```python
from build123d import *

# Parameters (mm, degrees)
SKETCH1_W               = 19.05
SKETCH1_H               = 19.05
SKETCH1_W_2             = 15.875
SKETCH1_H_2             = 15.875
BOSS_EXTRUDE1_DEPTH     = 196.85
CUT_EXTRUDE1_DEPTH      = 198.310348816
CUT_EXTRUDE1_DEPTH_BACK = 198.310348816
SKETCH2_R               = 6.35
SKETCH3_R               = 2.5
CUT_EXTRUDE2_DEPTH      = 30
SKETCH4_R               = 2.38125
CUT_EXTRUDE3_DEPTH      = 30


with BuildPart() as part:
    # Sketch1 → Boss-Extrude1 (new, symmetric)
    with BuildSketch(Plane.XY):
        Rectangle(SKETCH1_W, SKETCH1_H)
        Rectangle(SKETCH1_W_2, SKETCH1_H_2, mode=Mode.SUBTRACT)
    extrude(amount=BOSS_EXTRUDE1_DEPTH, both=True)

    # Sketch2 → Cut-Extrude1 (cut, two sides: drawn at the far end of the back side and taken through both)
    with BuildSketch(Plane(origin=(0, 0, 0), x_dir=(0, 0, -1), z_dir=(1, 0, 0)).offset(-CUT_EXTRUDE1_DEPTH_BACK)):
        Circle(SKETCH2_R)
    extrude(amount=CUT_EXTRUDE1_DEPTH + CUT_EXTRUDE1_DEPTH_BACK, mode=Mode.SUBTRACT)

    # Sketch3 → Cut-Extrude2 (cut)
    with BuildSketch(Plane(origin=(-152.4, 13.525, 0), x_dir=(1, 0, 0), z_dir=(0, 1, 0))):
        with Locations(Location((152.4, -186.375, 0), (0, 0, 270))):
            Circle(SKETCH3_R)
        with Locations(Location((152.4, -166.375, 0), (0, 0, 270))):
            Circle(SKETCH3_R)
    cut_extrude2 = extrude(amount=-CUT_EXTRUDE2_DEPTH, mode=Mode.SUBTRACT)

    # Mirror1: Cut-Extrude2 across Front Plane
    add(cut_extrude2.mirror(Plane.XY), mode=Mode.SUBTRACT)

    # Sketch4 → Cut-Extrude3 (cut)
    with BuildSketch(Plane(origin=(-152.4, 18.1864, 0), x_dir=(1, 0, 0), z_dir=(0, 1, 0))):
        with Locations(Location((152.4, -127, 0), (0, 0, 270))):
            Circle(SKETCH4_R)
        with Locations(Location((152.4, 127, 0), (0, 0, 270))):
            Circle(SKETCH4_R)
        with Locations(Location((152.4, -50.8, 0), (0, 0, 270))):
            Circle(SKETCH4_R)
        with Locations(Location((152.4, 50.8, 0), (0, 0, 270))):
            Circle(SKETCH4_R)
    extrude(amount=-CUT_EXTRUDE3_DEPTH, mode=Mode.SUBTRACT)


solid = part.part
```
Input: part model. Units: mm. Frame: model coordinates. A direction names the side the tool comes from. Coordinates: 2 decimals unless noted, no trailing zeros.
Q1. Mould query, pull axis Y, two halves, no side actions, for faces 1 (the flat face through (9.525, 6, 3)), 2 (the flat face through (0, 9.525, 3)), 3 (the cylindrical face through (8.72, -6.2, 1.38)). Classes: +Y half, -Y half, draft (parallel to the pull), parting line (faces both ways), or undercut.
Results are:
face 1: draft
face 2: +Y half
face 3: undercut
Q2. Contact query for a flat-ended pin moving along its axis: pin 1 (3 mm diameter, centred on x = 0, z = -166.375, fed in from -Y). Output: stop coordinate, or through.
Results are:
pin 1: passes through
Q3. Line query: line 1 along X through (y, z) = (-5.25, 98.5) (1 decimal); line 2 along X through (y, z) = (-8.4, 127) (3 decimals). Output: solid intervals per line, ascending.
Results are:
line 1: x = -9.5 to -7.9, 7.9 to 9.5
line 2: x = -9.525 to -2.381, 2.381 to 9.525
Q4. Set-up query: faces 4 (the flat face through (-7.938, 7, 3)), 5 (the flat face through (-9, 0, -196.85)). Return all of +Z, -Z, +X, -X, +Y, -Y with unobstructed straight access to the full face (end or side cutting, diameter ignored); none if empty.
Results are:
face 4: +Z, -Z
face 5: -Z, +X, -X, +Y, -Y
Q5. Section A-A, the plane y = 0. Give the number of separate pieces and of enclosed holes in the cut face, and give its area (3 significant figures).
Results are:
separate pieces: 4
enclosed holes: 0
area: 1,210 mm2
